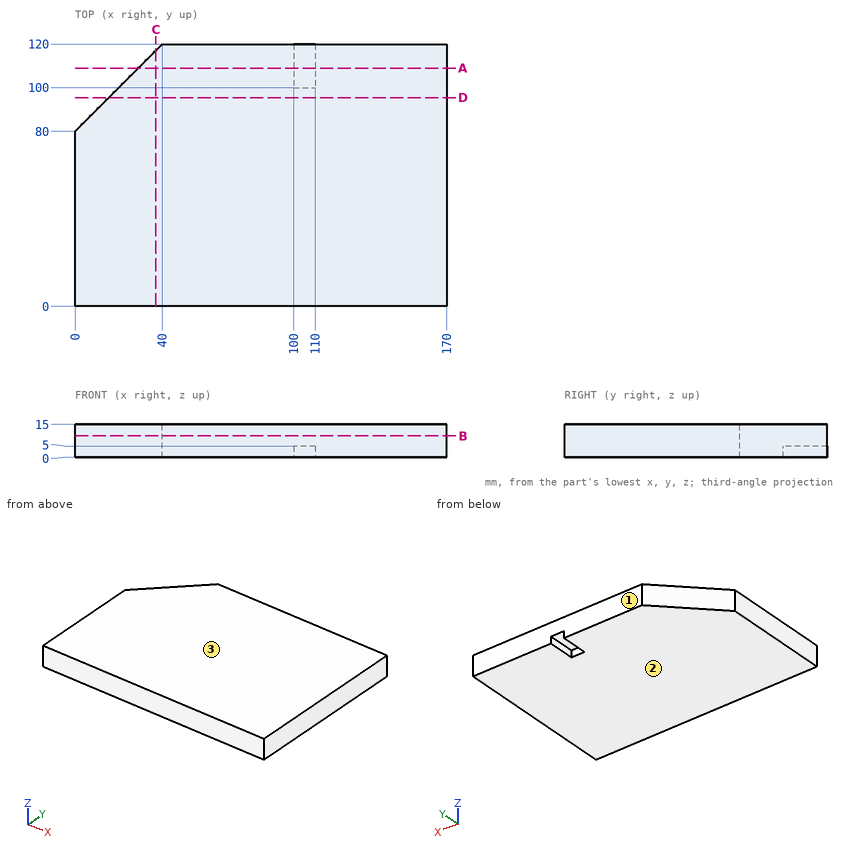
Geometry: see drawing. Coordinates: mm, zero at the bounding-box minimum. Give positions to 0.01 mm unless a question says otherwise; leave off trailing zeros. Order: outer loops, then holes, each group sorted by start corner. A loop starts at its lowest first (then second) coordinate and runs counter-clockwise, first axis right, second up. Notation, with made-up numbers: (82.25, -22) - (102.25, -22) arc R27 cw to (102.25, -3) - close; hole circle Ø3 at (32.5, 59). An arc over 180 degrees is marked (long way). One line per item, written item: value.
1. Cut plane C-C, the plane x = 37. Output: boundary loops of the cut face in (y, z), and give its area (4 significant figures).
Determined:
outline: (0, 0) - (117, 0) - (117, 15) - (0, 15) - close
area: 1,755 mm2
2. Draft query along Z for the marked faces 1, 2 and 3. Return one class per face: released by +Z, released by -Z, zero draft, split by the parting line, or undercut.
Determined:
face 1: zero draft
face 2: released by -Z
face 3: released by +Z
3. Cut plane B-B, the plane z = 9.75. Output: boundary loops of the cut face in (x, y), and give its area (3 significant figures).
Determined:
outline: (0, 0) - (170, 0) - (170, 120) - (40, 120) - (0, 80) - close
area: 19,600 mm2
4. Cut plane A-A, the plane y = 109. Output: boundary loops of the cut face in (x, z).
Determined:
outline: (29, 0) - (100, 0) - (100, 5) - (110, 5) - (110, 0) - (170, 0) - (170, 15) - (29, 15) - close
5. Cut plane D-D, the plane y = 95.5. Output: boundary loops of the cut face in (x, z), and give its area (3 significant figures).
Determined:
outline: (15.5, 0) - (170, 0) - (170, 15) - (15.5, 15) - close
area: 2,320 mm2
6. Pin query (flat end, axial travel): pin 1 Ø6 at (x, z) = (48.5, 12.5) entering from -Y; pin 2 Ø5 at (x, y) = (106.5, 106) entering from -Z; pin 3 Ø4 at (y, z) = (105.5, 2) entering from -X. Return the tip coordinate at first contact, or that it passes through.
Determined:
pin 1: y = 0
pin 2: z = 5
pin 3: x = 23.5
7. Line query: probe 1 along X at (y, z) = (112, 12); probe 2 along X at (y, z) = (96.5, 6.25); probe 3 along Y at (x, z) = (18.5, 7.5). Output: solid intervals per line, ascending.
Determined:
probe 1: 32 to 170
probe 2: 16.5 to 170
probe 3: 0 to 98.5
